Verification items for the finished model (mm, model axes). Face numbers are marked on the shaded views. A direction names the side the tool comes from. Coordinates: 2 decimals unless noted, no trailing zeros. Write each loop counter-clockwise with the first axis right and the second up, starting at its lowest first coordinate (ties: lowest second). Pieces come first, ordered by that corner, then holes. Notation, with made-up numbers: M 50,76.5 L 58,76.5 A25 cw 58,103.5 Z; hole C 37.5,70 d3. An arc over 180 degrees is marked long. One line per item, written item: value.
```python
from build123d import *

# Parameters (mm, degrees)
F0_R             = 40
F1_DEPTH         = 8
F2_R             = 9.5
F3_DEPTH         = 8.001
F5_R             = 3.25
F6_DEPTH         = 4
F8_DEPTH         = 5
F9_R             = 3.25
F10_DEPTH        = 2
F12_R            = 2
F13_DEPTH        = 15
F13_COPIES_COUNT = 4


# Not quite as in the source:
# - a pattern or mirror of a feature is missing from the dataset's text; its kind, count and spacing are read off the source's solid


with BuildPart() as f1:
    # F0 (on Top) → F1 (new body)
    with BuildSketch(Plane.XY):
        Circle(F0_R)
    extrude(amount=F1_DEPTH)

    # F2 (on face) → F3 (cut, through all)
    with BuildSketch(Plane.XY.offset(8)):
        Circle(F2_R)
    extrude(amount=-F3_DEPTH, mode=Mode.SUBTRACT)

    # F5 (on face) → F6 (cut)
    with BuildSketch(Plane.XY.offset(8)):
        with Locations((14.5, 0)):
            Circle(F5_R)
    extrude(amount=-F6_DEPTH, mode=Mode.SUBTRACT)

    # F7 (on face) → F8 (cut)
    with BuildSketch(Plane.XY.offset(8)):
        with BuildLine():
            Line((-17.75, 3.25), (-17.75, -3.5))
            ThreePointArc((-17.75, -3.5), (-14.5, -6.75), (-11.25, -3.5))
            Line((-11.25, -3.5), (-11.25, 3.25))
            ThreePointArc((-11.25, 3.25), (-14.5, 6.5), (-17.75, 3.25))
        make_face()
    extrude(amount=-F8_DEPTH, mode=Mode.SUBTRACT)

    # F9 (on face) → F10 (cut)
    with BuildSketch(Plane.XY.offset(8)):
        with Locations((0, -20.4880452948)):
            Circle(F9_R)
    extrude(amount=-F10_DEPTH, mode=Mode.SUBTRACT)

    # F12 (on offset) → F13 (cut)
    with BuildSketch(Plane.XZ.offset(40.792)):
        with Locations((0, 4)):
            Circle(F12_R)
    f13 = extrude(amount=-F13_DEPTH, mode=Mode.SUBTRACT)

    # F13_copies: F13 ×4 about axis
    f13_copies_axis = Axis((0, 0, 0), (0, 0, 1))
    for i in range(1, F13_COPIES_COUNT):
        add(f13.rotate(f13_copies_axis, i * 360 / F13_COPIES_COUNT), mode=Mode.SUBTRACT)


solid = f1.part
```
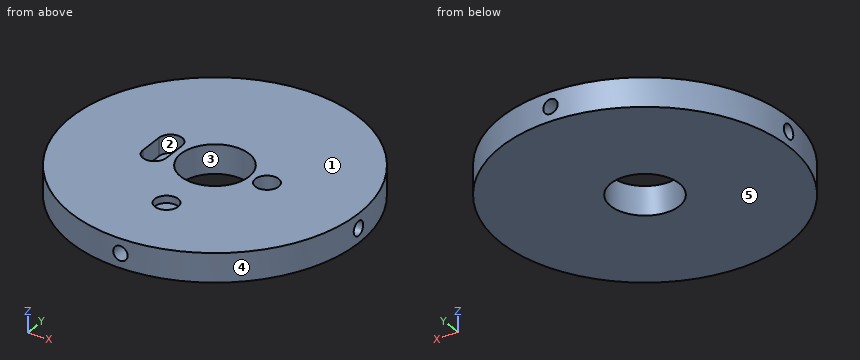
Item 1: Access from +Z, -Z, +X, -X, +Y, -Y to the whole of each face (thin tool, end or side, straight path). Record for the marked faces 1 and 2.
The answers:
face 1: +Z, +X, -X, +Y, -Y
face 2: +Z
Item 2: Cross-section at A-A, the plane y = 0. Enter the section's corners in (x, z), and give its area (3 significant figures).
The answers:
outline: M -40,0 L -9.5,0 L -9.5,8 L -11.25,8 L -11.25,3 L -17.75,3 L -17.75,8 L -40,8 L -40,6 L -25.79,6 L -25.79,2 L -40,2 Z; M 9.5,0 L 40,0 L 40,2 L 25.79,2 L 25.79,6 L 40,6 L 40,8 L 17.75,8 L 17.75,4 L 11.25,4 L 11.25,8 L 9.5,8 Z
area: 316 mm²
Item 3: Cross-section at C-C, the plane y = -27. Enter the section's corners in (x, z).
The answers:
outline: M -29.51,0 L 29.51,0 L 29.51,8 L -29.51,8 Z; hole C 0,4 d4
Item 4: Cross-section at D-D, the plane x = 13.5. Enter the section's corners in (y, z).
The answers:
outline: M -37.65,0 L 37.65,0 L 37.65,8 L 3.09,8 L 3.09,4 L -3.09,4 L -3.09,8 L -37.65,8 Z
Item 5: Draft check along Y on the marked faces 3, 4 and 5. Enter one of: released by +Y, released by -Y, zero draft, split by the parting line, or undercut.
The answers:
face 3: undercut
face 4: split by the parting line
face 5: zero draft
Item 6: Cross-section at B-B, the plane x = 0. Enter the section's corners in (y, z).
The answers:
outline: M -40,0 L -9.5,0 L -9.5,8 L -17.24,8 L -17.24,6 L -23.74,6 L -23.74,8 L -40,8 L -40,6 L -25.79,6 L -25.79,2 L -40,2 Z; M 9.5,0 L 40,0 L 40,2 L 25.79,2 L 25.79,6 L 40,6 L 40,8 L 9.5,8 Z
Item 7: Go/stop test with flat-tipped pins: P1, Ø2, axis at x = -0.5, y = -22, coming from the +Z side; P2, Ø1.5, axis at y = 0.5, z = 2.5, coming from the +X side; P3, Ø3, axis at x = 0, z = 4, coming from the +Y side; P4, Ø3, axis at y = -27.5, z = 3.5, coming from the +X side. Record where each tip stops, or that it passes through.
The answers:
P1: stops at z = 6
P2: stops at x = 40
P3: stops at y = 25.79
P4: stops at x = 30.4
Item 8: Scan lines: line 1 (Y direction, x = 0, z = 7.6); line 2 (Z direction, x = 36.5, y = 0); line 3 (X direction, y = -33.5, z = 5.75). Record each from-to range of solid material in increasing order.
The answers:
line 1: y = -40 to -23.74, -17.24 to -9.5, 9.5 to 40
line 2: z = 0 to 2, 6 to 8
line 3: x = -21.86 to -0.97, 0.97 to 21.86
